from build123d import *

# Parameters (mm, degrees)
F2_R = 5
F3_T = -1


with BuildPart() as f1:
    # F0 (on Front) → F1 (revolve)
    with BuildSketch(Plane.XZ):
        Polygon((0, 120), (-35, 120), (-54.2100556195, 51.1340316432), (-51.4871776104, 27.2081736475), (-40.1005893946, 16.3166560233), (-23.8004934928, 11.769769421), (-3.6637331643, 1.811781532), (0, 0), align=None)
        Polygon((0, -102.4070009589), (0, 0), (-3.6637331643, 1.811781532), (-3.6637331643, -88.188218468), (-36.5668833256, -102.4070009589), align=None)
    revolve(axis=Axis((0, 0, 8.7964995205), (0, 0, -1)))

    # F2
    f2_edges = [f1.edges().sort_by_distance(p)[0] for p in [
        (3.663733, 0, 1.811782),
        (3.663733, 0, -88.188218),
    ]]
    fillet(f2_edges, radius=F2_R)

    # F3
    f3_openings = [f1.faces().sort_by_distance(p)[0] for p in [
        (0, 0, 120),
    ]]
    offset(amount=F3_T, openings=f3_openings, kind=Kind.INTERSECTION)


solid = f1.part
Model file for the job. Use its own axes, mm. A direction names the side the tool comes from. Round coordinates to 2 decimals unless told otherwise and drop trailing zeros. Order: outer loops, then holes, each group sorted by start corner. A loop starts at its lowest first (then second) coordinate and runs counter-clockwise, first axis right, second up.
(1) Drill centre lines: line 1 (X direction, y = 0, z = -59); line 2 (Z direction, x = -16.5, y = 9). Where is each one in solid material? Low to high.
(2) Band-saw the part on C-C (z = 70.5). List the corners of the cut face in (x, y), then the cut area to 3 significant figures.
(3) Pin check, flat tips, straight feed: pin 1 (8 mm diameter, centred on x = 4.5, y = -8, fed in from +Z); pin 2 (4 mm diameter, centred on x = -21.5, z = 67, fed in from -Y); pin 3 (2 mm diameter, centred on x = 34.5, y = -39, fed in from -Z). Stop position of each tip, or through.
(4) Pull direction X, two halves, no side cores. Call faces 4 (the face through (11.111, -50.036, 34.009)), 5 (the face through (1, 1, -102.407)), 6 (the face through (5.29, 40.31, 16.85)): released by +X, released by -X, zero draft, split by the parting line, or undercut.
(5) 3-axis set-ups, long thin cutter, end or side, ignore diameter. For faces 1 (the face through (19.52, -14.96, 11.99)), 2 (the face through (-29, 18, 120)), 3 (the face through (-2.46, -1.02, -43.68)): which of +Z, -Z, +X, -X, +Y, -Y reach the whole face in a straight line?
(6) Band-saw the part on B-B (z = -71). List the corners of the cut face in (x, y).
(7) Band-saw the part on A-A (x = -12). Give the number of separate pieces and of enclosed holes in the cut face, then the cut area to 3 significant figures.
Verdict:
1. line 1: x = -3.66 to -2.66, 2.66 to 3.66
1. line 2: z = -102.41 to -101.41, -95.82 to -94.73, 9.29 to 10.41
2. outline: circle Ø97.62 at (0, 0); hole circle Ø95.54 at (0, 0)
2. area: 315 mm2
3. pin 1: stops at z = 7.63
3. pin 2: stops at y = -46
3. pin 3: stops at z = 26.81
4. face 4: undercut
4. face 5: zero draft
4. face 6: split by the parting line
5. face 1: none
5. face 2: +Z, +X, -X, +Y, -Y
5. face 3: +Z
6. outline: circle Ø7.33 at (0, 0); hole circle Ø5.33 at (0, 0)
7. separate pieces: 2
7. enclosed holes: 1
7. area: 446 mm2
